Check sheet for the modelled part. Datum: model origin and axes. Units: mm. Face numbers are marked on the shaded views. A direction names the side the tool comes from. Round coordinates to 2 decimals unless told otherwise and drop trailing zeros. Order: outer loops, then holes, each group sorted by start corner. A loop starts at its lowest first (then second) coordinate and runs counter-clockwise, first axis right, second up. Notation, with made-up numbers: (68, 52.5) -> (92, 52.5) arc R20 cw to (92, 87.5) -> close; hole circle Ø10 at (42.25, 25.5). An arc over 180 degrees is marked (long way). Answer in a Markdown table with one row per item.
```python
from build123d import *

# Parameters (mm, degrees)
SKETCH1_W           = 13.0048
SKETCH1_H           = 14.224
SKETCH1_R           = 0.508
SKETCH1_R_2         = 1.5
BOSS_EXTRUDE1_DEPTH = 1.6383
SKETCH2_W           = 7.5
SKETCH2_H           = 6
BOSS_EXTRUDE3_DEPTH = 2.3876


with BuildPart() as part:
    # Sketch1 → Boss-Extrude1 (new body)
    with BuildSketch(Plane(origin=(0, 0, 0), x_dir=(1, 0, 0), z_dir=(0, 1, 0))):
        with Locations((6.5024, 7.112)):
            Rectangle(SKETCH1_W, SKETCH1_H)
        with Locations((1.4224, 13)):
            Circle(SKETCH1_R, mode=Mode.SUBTRACT)
        with Locations((3.9624, 13)):
            Circle(SKETCH1_R, mode=Mode.SUBTRACT)
        with Locations((6.5024, 13)):
            Circle(SKETCH1_R, mode=Mode.SUBTRACT)
        with Locations((9.0424, 13)):
            Circle(SKETCH1_R, mode=Mode.SUBTRACT)
        with Locations((11.5824, 13)):
            Circle(SKETCH1_R, mode=Mode.SUBTRACT)
        with Locations((2.0828, 6.9)):
            Circle(SKETCH1_R_2, mode=Mode.SUBTRACT)
        with Locations((10.922, 6.9)):
            Circle(SKETCH1_R_2, mode=Mode.SUBTRACT)
    extrude(amount=BOSS_EXTRUDE1_DEPTH)

    # Sketch2 → Boss-Extrude3 (add)
    with BuildSketch(Plane(origin=(0, 1.6383, 0), x_dir=(1, 0, 0), z_dir=(0, 1, 0))):
        with Locations((6.5024, 2.4356)):
            Rectangle(SKETCH2_W, SKETCH2_H)
    extrude(amount=BOSS_EXTRUDE3_DEPTH)


solid = part.part
```
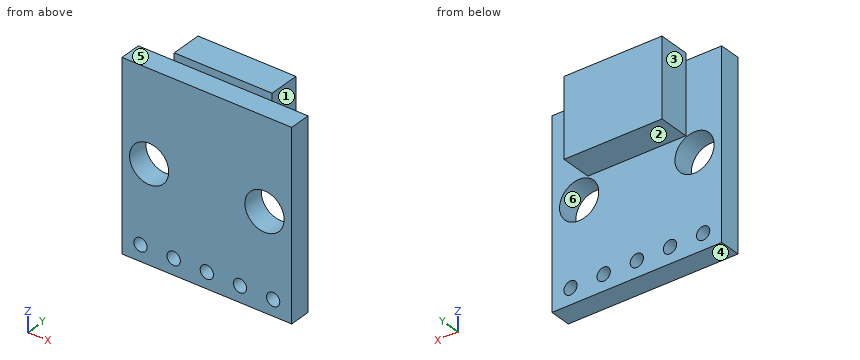
(1) Section check C-C on y = 1.4. Record the boundary of the cut face in (x, z), plus the area to 3 significant figures.
Solutions:
| item | result |
|---|---|
| outline | (0, -14.22) -> (13, -14.22) -> (13, 0) -> (0, 0) -> close; hole circle Ø3 at (2.08, -6.9); hole circle Ø1.02 at (1.42, -13); hole circle Ø1.02 at (3.96, -13); hole circle Ø1.02 at (6.5, -13); hole circle Ø1.02 at (9.04, -13); hole circle Ø3 at (10.92, -6.9); hole circle Ø1.02 at (11.58, -13) |
| area | 167 mm^2 |
(2) Section check A-A on z = -6.9. Record the boundary of the cut face in (x, y), plus the area to 3 significant figures.
Solutions:
| item | result |
|---|---|
| outline | (0, 0) -> (0.58, 0) -> (0.58, 1.64) -> (0, 1.64) -> close; (3.58, 0) -> (9.42, 0) -> (9.42, 1.64) -> (3.58, 1.64) -> close; (12.42, 0) -> (13, 0) -> (13, 1.64) -> (12.42, 1.64) -> close |
| area | 11.5 mm^2 |
(3) Section check B-B on z = -13. Record the boundary of the cut face in (x, y), plus the area to 3 significant figures.
Solutions:
| item | result |
|---|---|
| outline | (0, 0) -> (0.91, 0) -> (0.91, 1.64) -> (0, 1.64) -> close; (1.93, 0) -> (3.45, 0) -> (3.45, 1.64) -> (1.93, 1.64) -> close; (4.47, 0) -> (5.99, 0) -> (5.99, 1.64) -> (4.47, 1.64) -> close; (7.01, 0) -> (8.53, 0) -> (8.53, 1.64) -> (7.01, 1.64) -> close; (9.55, 0) -> (11.07, 0) -> (11.07, 1.64) -> (9.55, 1.64) -> close; (12.09, 0) -> (13, 0) -> (13, 1.64) -> (12.09, 1.64) -> close |
| area | 13.0 mm^2 |
(4) Depth check by flat-ended pin: pin 1 Ø1.2 at (y, z) = (3, -4) entering from -X; pin 2 Ø0.8 at (x, y) = (7, 1) entering from +Z; pin 3 Ø6.5 at (x, z) = (3.5, -9.5) entering from +Y. Enter the tip coordinate at first touch or a pass-through.
Solutions:
| item | result |
|---|---|
| pin 1 | x = 2.75 |
| pin 2 | z = 0 |
| pin 3 | y = 1.64 |
(5) Draft check along Z on the marked faces 4, 5 and 6. Enter one of: pulls with the +Z half, pulls with the -Z half, needs draft (parallel to the pull), parting line crosses it, or undercut.
Solutions:
| item | result |
|---|---|
| face 4 | pulls with the -Z half |
| face 5 | pulls with the +Z half |
| face 6 | undercut |
(6) Section check D-D on x = 5. Record the boundary of the cut face in (y, z), plus the area to 3 significant figures.
Solutions:
| item | result |
|---|---|
| outline | (0, -14.22) -> (1.64, -14.22) -> (1.64, -5.44) -> (4.03, -5.44) -> (4.03, 0.56) -> (1.64, 0.56) -> (1.64, 0) -> (0, 0) -> close |
| area | 37.6 mm^2 |
(7) Scan lines: probe 1 along X at (y, z) = (0.95, -13); probe 2 along X at (y, z) = (1.25, -6.9); probe 3 along Z at (x, y) = (12, 0.3). Record each from-to range of solid material in increasing order. Write a range as from..to.
Solutions:
| item | result |
|---|---|
| probe 1 | 0..0.91, 1.93..3.45, 4.47..5.99, 7.01..8.53, 9.55..11.07, 12.09..13 |
| probe 2 | 0..0.58, 3.58..9.42, 12.42..13 |
| probe 3 | -14.22..-13.29, -12.71..-7.94, -5.86..0 |
(8) Tool access check on the marked faces 1, 2 and 3. Record the directions out of +Z, -Z, +X, -X, +Y, -Y that give a thin tool (end or side, any length) a straight path to the whole face; none if there is none.
Solutions:
| item | result |
|---|---|
| face 1 | +Z, -Z, +X, +Y |
| face 2 | -Z, +X, -X, +Y |
| face 3 | +Z, -Z, -X, +Y |
